from build123d import *

# Parameters (mm, degrees)
SKETCH1_R      = 3.9878
EXTRUDE1_DEPTH = 4.7752
FILLET1_R      = 3.175
EXTRUDE2_DEPTH = 3.9624


with BuildPart() as part:
    # Sketch1 → Extrude1 (new body)
    with BuildSketch(Plane.XY):
        with BuildLine():
            Line((9.832512944, 1.076805598), (41.582512944, 1.076805598))
            ThreePointArc((41.582512944, 1.076805598), (43.827576974, 2.006741568), (44.757512944, 4.251805598))
            Line((44.757512944, 4.251805598), (44.757512944, 36.001805598))
            ThreePointArc((44.757512944, 36.001805598), (43.827576974, 38.246869628), (41.582512944, 39.176805598))
            Line((41.582512944, 39.176805598), (9.832512944, 39.176805598))
            ThreePointArc((9.832512944, 39.176805598), (7.587448914, 38.246869628), (6.657512944, 36.001805598))
            Line((6.657512944, 36.001805598), (6.657512944, 4.251805598))
            ThreePointArc((6.657512944, 4.251805598), (7.587448914, 2.006741568), (9.832512944, 1.076805598))
        make_face()
        with Locations((25.707512944, 20.126805598)):
            Circle(SKETCH1_R, mode=Mode.SUBTRACT)
    extrude(amount=EXTRUDE1_DEPTH)

    # Fillet1
    fillet1_edges = [part.edges().sort_by_distance(p)[0] for p in [
        (25.707512944, 1.076805598, 4.7752),
        (43.827576974, 2.006741568, 4.7752),
        (44.757512944, 20.126805598, 4.7752),
        (43.827576974, 38.246869628, 4.7752),
        (25.707512944, 39.176805598, 4.7752),
        (7.587448914, 38.246869628, 4.7752),
        (6.657512944, 20.126805598, 4.7752),
        (7.587448914, 2.006741568, 4.7752),
    ]]
    fillet(fillet1_edges, radius=FILLET1_R)

    # Sketch2 → Extrude2 (add)
    with BuildSketch(Plane(origin=(0, 0, 0), x_dir=(-1, 0, 0), z_dir=(0, 0, -1))):
        with BuildLine():
            Line((-29.339712944, 35.214405598), (-22.075312944, 35.214405598))
            ThreePointArc((-22.075312944, 35.214405598), (-21.80590526, 35.325997914), (-21.694312944, 35.595405598))
            Line((-21.694312944, 35.595405598), (-21.694312944, 38.795805598))
            ThreePointArc((-21.694312944, 38.795805598), (-21.80590526, 39.065213281), (-22.075312944, 39.176805598))
            Line((-22.075312944, 39.176805598), (-29.339712944, 39.176805598))
            ThreePointArc((-29.339712944, 39.176805598), (-29.609120627, 39.065213281), (-29.720712944, 38.795805598))
            Line((-29.720712944, 38.795805598), (-29.720712944, 35.595405598))
            ThreePointArc((-29.720712944, 35.595405598), (-29.609120627, 35.325997914), (-29.339712944, 35.214405598))
        make_face()
    extrude(amount=EXTRUDE2_DEPTH)


solid = part.part
Could you check a few things on this model? Use its own coordinates, in mm. A direction names the side the tool comes from. Coordinates: 2 decimals unless noted, no trailing zeros. Write each loop counter-clockwise with the first axis right and the second up, starting at its lowest first coordinate (ties: lowest second). Pieces come first, ordered by that corner, then holes. Notation, with made-up numbers: M 72,-9.75 L 118,-9.75 A5 cw 118,-2.75 Z; hole C -11.75,72.25 d4. An arc over 180 degrees is marked long. One line per question, with ' | ' between items.
1) Imagine slicing it at C-C, the plane z = 3. Write out the boundary of the cut face in (x, y), and give its area (3 significant figures).
Checks:
outline: M 6.98,4.25 A2.85 ccw 9.83,1.4 L 41.58,1.4 A2.85 ccw 44.43,4.25 L 44.43,36 A2.85 ccw 41.58,38.85 L 9.83,38.85 A2.85 ccw 6.98,36 Z; hole C 25.71,20.13 d7.98 | area: 1,350 mm²
2) For faces 1 (the face through (21.694, 37, -2)), 2 (the face through (29.721, 37, -2)), 3 (the face through (26, 35.214, -2)), which set-ups out of +Z, -Z, +X, -X, +Y, -Y let a thin tool reach every point of the face, with its end or its side?
Checks:
face 1: -Z, -X, +Y, -Y | face 2: -Z, +X, +Y, -Y | face 3: -Z, +X, -X, -Y
3) Imagine slicing it at B-B, the plane y = 19. Write out the boundary of the cut face in (x, z) (3 decimals), and give its area (3 significant figures).
Checks:
outline: M 6.658,0 L 21.882,0 L 21.882,4.775 L 9.833,4.775 A3.175 ccw 6.658,1.6 Z; M 29.533,0 L 44.758,0 L 44.758,1.6 A3.175 ccw 41.583,4.775 L 29.533,4.775 Z | area: 141 mm²
4) Imagine slicing it at D-D, the plane x = 18. Write out the boundary of the cut face in (y, z) (3 decimals), and give its area (3 significant figures).
Checks:
outline: M 1.077,0 L 39.177,0 L 39.177,1.6 A3.175 ccw 36.002,4.775 L 4.252,4.775 A3.175 ccw 1.077,1.6 Z | area: 178 mm²
5) I need wall thicknesses on probe 1 along Z at (x, y) = (16, 5.5); probe 2 along Y at (x, z) = (25, 2); probe 3 along Z at (x, y) = (14.5, 36.5). Which ranges of each line are inside material? Lowest first, please. Write a range as [from, to].
Checks:
probe 1: [0, 4.78] | probe 2: [1.1, 16.2], [24.05, 39.15] | probe 3: [0, 4.74]
6) For pin 1 Ø2 at (x, z) = (25.5, -1.5) entering from -Y; pin 2 Ø1.6 at (y, z) = (37, -2.5) entering from -X; pin 3 Ø2.5 at (y, z) = (37, -2) entering from +X, each with a flat end and sliding along its axis, tell me the tip position at first contact or that it passes through.
Checks:
pin 1: y = 35.21 | pin 2: x = 21.69 | pin 3: x = 29.72
7) If we mould it in two halves opening along X, with no side actions, what happens to faces 4 (the face through (29.39, 18.6, 2.35)), 5 (the face through (44.758, 20, 1)), 6 (the face through (29, 24, 4.775))? For each: released by +X, released by -X, zero draft, split by the parting line, or undercut.
Checks:
face 4: undercut | face 5: released by +X | face 6: zero draft
8) Imagine slicing it at A-A, the plane x = 28.5. Write out the boundary of the cut face in (y, z) (3 decimals).
Checks:
outline: M 1.077,0 L 17.28,0 L 17.28,4.775 L 4.252,4.775 A3.175 ccw 1.077,1.6 Z; M 22.974,0 L 35.214,0 L 35.214,-3.962 L 39.177,-3.962 L 39.177,1.6 A3.175 ccw 36.002,4.775 L 22.974,4.775 Z
